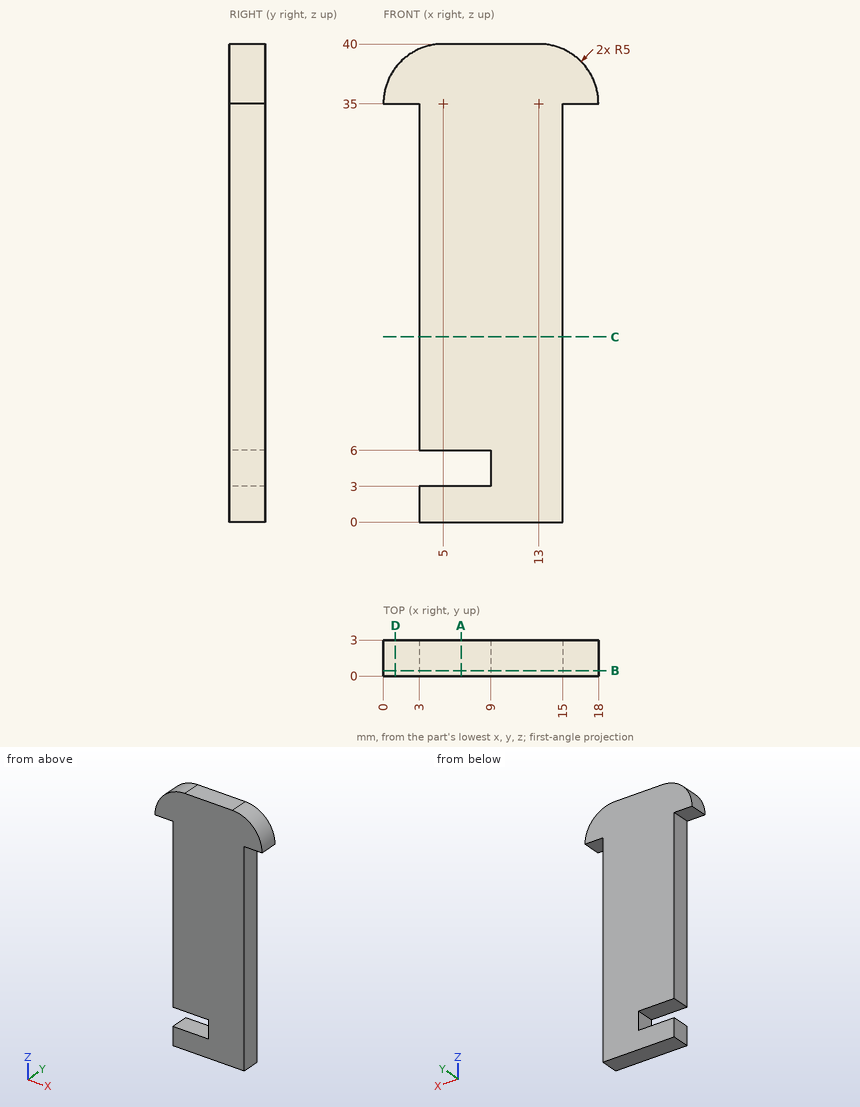
Geometry: see drawing. Coordinates: mm, zero at the bounding-box minimum. Give positions to 0.01 mm unless a question says otherwise; leave off trailing zeros. Order: outer loops, then holes, each group sorted by start corner. A loop starts at its lowest first (then second) coordinate and runs counter-clockwise, first axis right, second up. Notation, with made-up numbers: (-15, -1) -> (35, -1) arc R22 cw to (35, 25) -> close; hole circle Ø5 at (45.5, -26). An arc over 180 degrees is marked (long way). Write item = value, one per line.
Q1. Cut plane A-A, the plane x = 6.5. Output: boundary loops of the cut face in (y, z).
Data:
outline = (0, 0) -> (3, 0) -> (3, 3) -> (0, 3) -> close; (0, 6) -> (3, 6) -> (3, 40) -> (0, 40) -> close
Q2. Pin query (flat end, axial travel): pin 1 (1.5 mm diameter, centred on y = 2, z = 11.5, fed in from +X); pin 2 (1.5 mm diameter, centred on x = 16.5, y = 2, fed in from -Z); pin 3 (0.9 mm diameter, centred on y = 2, z = 18.5, fed in from -X). Return the tip coordinate at first contact, or that it passes through.
Data:
pin_1 = 15
pin_2 = 35
pin_3 = 3
Q3. Cut plane C-C, the plane z = 15.5. Output: boundary loops of the cut face in (x, y).
Data:
outline = (3, 0) -> (15, 0) -> (15, 3) -> (3, 3) -> close
Q4. Cut plane D-D, the plane x = 1. Output: boundary loops of the cut face in (y, z), and give its area (3 significant figures).
Data:
outline = (0, 35) -> (3, 35) -> (3, 38) -> (0, 38) -> close
area = 9.00 mm^2
Q5. Cut plane B-B, the plane y = 0.45. Output: boundary loops of the cut face in (x, z), and give its area (3 significant figures).
Data:
outline = (0, 35) -> (3, 35) -> (3, 6) -> (9, 6) -> (9, 3) -> (3, 3) -> (3, 0) -> (15, 0) -> (15, 35) -> (18, 35) arc R5 ccw to (13, 40) -> (5, 40) arc R5 ccw to start
area = 481 mm^2
Q6. Material intervals for line 1 (Z direction, x = 5.25, y = 1.15); line 2 (X direction, y = 1.15, z = 17.5); line 3 (Z direction, x = 13.25, y = 2.4), sorted ascending. Write a range as from..to.
Data:
line_1 = 0..3, 6..40
line_2 = 3..15
line_3 = 0..39.99
